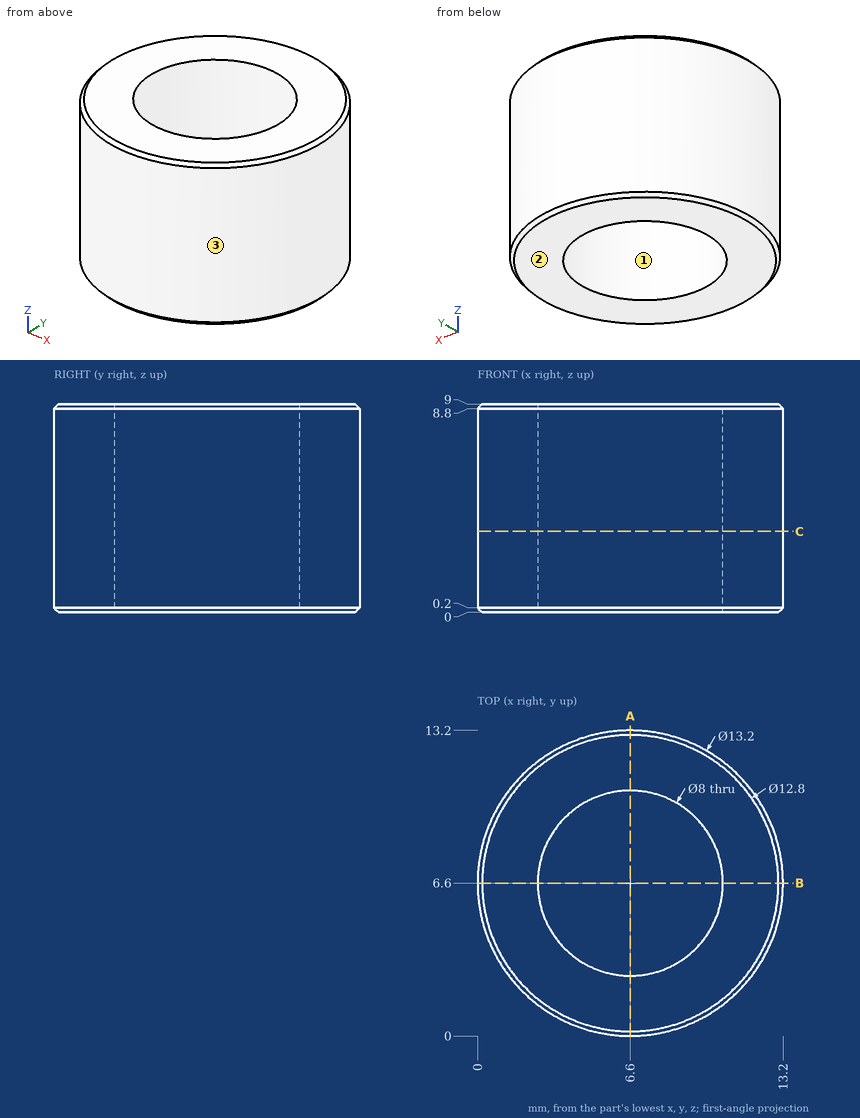
For this review, use the dimensioned drawing (mm, ordinates from the lowest corner) and the shaded views. Round coordinates to 2 decimals unless told otherwise and drop trailing zeros. Write each loop counter-clockwise with the first axis right and the second up, starting at its lowest first coordinate (ties: lowest second). Pieces come first, ordered by that corner, then holes. Notation, with made-up numbers: (-9, -1) - (10, -1) arc R27 cw to (10, 29) - close; hole circle Ø3 at (9, 17.5). An arc over 180 degrees is marked (long way). Use a Markdown table: item, result.
Q1. We need section C-C (z = 3.5). Give the boundary of the cut face in (x, y).
Derived:
| item | result |
|---|---|
| outline | circle Ø13.2 at (6.6, 6.6); hole circle Ø8 at (6.6, 6.6) |
Q2. Wall thickness on line 1 along Y through (x, z) = (6.6, 4.5); line 2 along Y through (x, z) = (4, 2.25); line 3 along X through (y, z) = (3.5, 2.75): over which ranges is each line inside the solid? List them lowest first.
Derived:
| item | result |
|---|---|
| line 1 | y = 0 to 2.6, 10.6 to 13.2 |
| line 2 | y = 0.53 to 3.56, 9.64 to 12.67 |
| line 3 | x = 0.77 to 4.07, 9.13 to 12.43 |
Q3. Clearance check with flat-ended pins moving along their axes: pin 1 (4 mm diameter, centred on x = 10.5, z = 2.5, fed in from -Y); pin 2 (4 mm diameter, centred on x = 5.5, z = 6, fed in from -Y); pin 3 (4 mm diameter, centred on x = 3.5, z = 2.5, fed in from +Y). State where each tip first meets the part, or that it passes through.
Derived:
| item | result |
|---|---|
| pin 1 | stops at y = 0.28 |
| pin 2 | stops at y = 0 |
| pin 3 | stops at y = 13.11 |
Q4. We need section A-A (x = 6.6). Give the boundary of the cut face in (y, z).
Derived:
| item | result |
|---|---|
| outline | (0, 0.2) - (0.2, 0) - (2.6, 0) - (2.6, 9) - (0.2, 9) - (0, 8.8) - close; (10.6, 0) - (13, 0) - (13.2, 0.2) - (13.2, 8.8) - (13, 9) - (10.6, 9) - close |
Q5. The part is to be moulded in two halves that separate along X. For the marked faces 1, 2 and 3, say which applies: pulls with the +X half, pulls with the -X half, needs draft (parallel to the pull), parting line crosses it, or undercut.
Derived:
| item | result |
|---|---|
| face 1 | undercut |
| face 2 | needs draft |
| face 3 | parting line crosses it |
